Here's how the part is built. I have some questions about the finished solid (model axes, mm). Face numbers are marked on the shaded views. A direction names the side the tool comes from. Give positions to 0.01 mm unless a question says otherwise; leave off trailing zeros.
Q1. I'm going to push flat-ended pins straight in: P1, Ø5, axis at x = -11.5, z = 2, coming from the +Y side; P2, Ø5, axis at y = -13.5, z = -2.5, coming from the -X side; P3, Ø6, axis at x = -19, z = 6, coming from the +Y side; P4, Ø4, axis at y = 7, z = -10, coming from the +X side. Where does each tip first touch, or does it pass through?
Q2. For the marked faces 1 and 2, which set-ups out of +Z, -Z, +X, -X, +Y, -Y let a thin tool reach every point of the face, with its end or its side?
Q3. Suppose I cut it at A-A (y = 0). Count the separate pieces of the cut face and the enclosed holes in it, and give its area (3 significant figures).
Q4. Thinking about a two-plate mould opening in Y: for the marked faces 3, 4 and 5, which applies, pulls with the +Y half, pulls with the -Y half, needs draft (parallel to the pull), parting line crosses it, or undercut?
Q5. I need wall thicknesses on probe 1 along Y at (x, z) = (-5.5, 13.5); probe 2 along Z at (x, y) = (-12.7, 14.5); probe 3 along X at (y, z) = (-7, 11). Which ranges of each line are inside material? Lowest first, please.
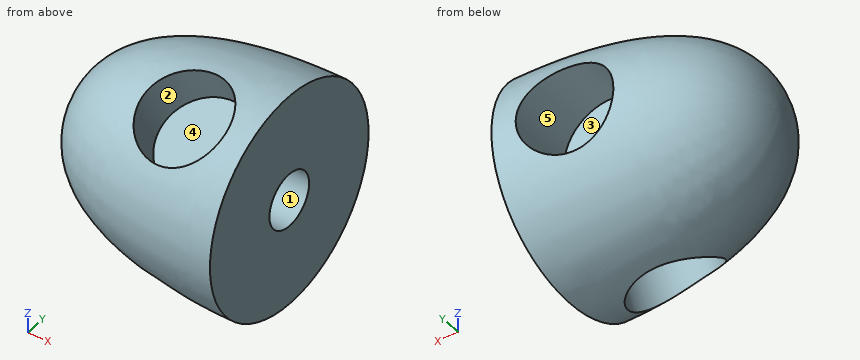
```python
from build123d import *

# Parameters (mm, degrees)
SKETCH2_R          = 5
CUT_EXTRUDE1_DEPTH = 12.7
SKETCH3_R          = 8.25
CUT_EXTRUDE2_DEPTH = 52.419937935
CIRPATTERN1_COUNT  = 3


with BuildPart() as part:
    # Sketch1 → Revolve1 (revolve)
    with BuildSketch(Plane.XY):
        with BuildLine():
            Line((0, 20), (0, 0))
            Line((0, 0), (-38.5, 0))
            add(Edge.make_bspline(
                [(-38.5, 0), (-38.5, 17.416386275), (-14.46163507, 20), (0, 20)],
                knots=[0, 0, 0, 0, 1, 1, 1, 1], degree=3))
        make_face()
    revolve(axis=Axis((0, 0, 0), (-1, 0, 0)))

    # Sketch2 → Cut-Extrude1 (cut)
    with BuildSketch(Plane(origin=(0, 0, 0), x_dir=(0, 0, -1), z_dir=(1, 0, 0))):
        Circle(SKETCH2_R)
    extrude(amount=-CUT_EXTRUDE1_DEPTH, mode=Mode.SUBTRACT)

    # Sketch3 → Cut-Extrude2 (cut, through all)
    with BuildSketch(Plane(origin=(0, 7.6, 0), x_dir=(1, 0, 0), z_dir=(0, 1, 0))):
        with Locations((-12.7, 0)):
            Circle(SKETCH3_R)
    cut_extrude2 = extrude(amount=CUT_EXTRUDE2_DEPTH, mode=Mode.SUBTRACT)

    # CirPattern1: Cut-Extrude2 ×3 about axis
    cirpattern1_axis = Axis((0, 0, 0), (1, 0, 0))
    for i in range(1, CIRPATTERN1_COUNT):
        add(cut_extrude2.rotate(cirpattern1_axis, i * 360 / CIRPATTERN1_COUNT), mode=Mode.SUBTRACT)


solid = part.part
```
Solutions:
1. P1: stops at y = 7.6
1. P2: stops at x = -33.78
1. P3: stops at y = 17.56
1. P4: stops at x = 0
2. face 1: +X
2. face 2: none
3. separate pieces: 1
3. enclosed holes: 2
3. area: 991 mm2
4. face 3: pulls with the +Y half
4. face 4: undercut
4. face 5: needs draft
5. probe 1: y = -14.58 to -12.45, -3.14 to 14.58
5. probe 2: z = -12.66 to -8.25, 8.25 to 12.66
5. probe 3: x = -31.58 to -20.93, -4.47 to 0
